```python
from build123d import *

# Parameters (mm, degrees)
F1_DEPTH       = 1.5
F2_DEPTH       = 10
F3_D           = 5
F3_CSINK_D     = 7
F3_CSINK_ANGLE = 90
F4_T1_DEPTH    = 36.6824583655
F4_T3_DEPTH    = 79.6824583655
F4_T5_DEPTH    = 19.5
F4_T7_DEPTH    = 47
F4_T13_DEPTH   = 52
F4_T17_DEPTH   = 24.5
F4_T24_DEPTH   = 24.5
F4_T28_DEPTH   = 52
F5_R           = 1


# Not quite as in the source:
# - a fillet or chamfer that OpenCascade refuses, or shapes differently, is made with other operations: its cross-section is extruded or revolved along the edge and cut away or added


with BuildPart() as f1:
    # F0 (on Front) → F1 (new body)
    with BuildSketch(Plane.XZ):
        Polygon((35, 27), (-35, 27), (-35, 0), (-25, 0), (-25, 16), (25, 16), (25, 0), (35, 0), align=None)
        Polygon((-25, 16), (-25, 0), (-23.5, 0), (-23.5, 14.5), (23.5, 14.5), (23.5, 0), (25, 0), (25, 16), align=None)
    extrude(amount=-F1_DEPTH)

    # F0 (on Front) → F2 (join)
    with BuildSketch(Plane.XZ):
        Polygon((-25, 16), (-25, 0), (-23.5, 0), (-23.5, 14.5), (23.5, 14.5), (23.5, 0), (25, 0), (25, 16), align=None)
    extrude(amount=-F2_DEPTH)

    # F3 (through all)
    with Locations(Plane.XZ):
        with Locations((28.6, 20.6), (-28.6, 20.6)):
            CounterSinkHole(F3_D / 2, F3_CSINK_D / 2, counter_sink_angle=F3_CSINK_ANGLE)

    # F4: fillet of radius 2 on 6 edges, made by hand

    # F4_s2 → F4_t1 (cut)
    with BuildSketch(Plane.XY.offset(-4.8412291828)):
        with BuildLine():
            ThreePointArc((-33.0635083269, 0), (-34.2882531983, 0.4188611699), (-35, 1.5))
            Line((-35, 1.5), (-35.0387298335, 1.49))
            ThreePointArc((-35.0387298335, 1.49), (-35.04, 0.75), (-35.04, 0))
            Line((-35.04, 0), (-35, -0.04))
            Line((-35, -0.04), (-33.0635083269, -0.04))
            Line((-33.0635083269, -0.04), (-33.0635083269, 0))
        make_face()
        with BuildLine():
            ThreePointArc((35, 1.5), (34.2882531983, 0.4188611699), (33.0635083269, 0))
            Line((33.0635083269, 0), (33.0635083269, -0.04))
            Line((33.0635083269, -0.04), (35, -0.04))
            Line((35, -0.04), (35.04, 0))
            ThreePointArc((35.04, 0), (35.04, 0.75), (35.0387298335, 1.49))
            Line((35.0387298335, 1.49), (35, 1.5))
        make_face()
    extrude(amount=F4_T1_DEPTH, mode=Mode.SUBTRACT)

    # F4_s4 → F4_t3 (cut)
    with BuildSketch(Plane.YZ.offset(-39.8412291828)):
        with BuildLine():
            ThreePointArc((1.5, 27), (0.4188611699, 26.2882531983), (0, 25.0635083269))
            Line((0, 25.0635083269), (-0.04, 25.0635083269))
            Line((-0.04, 25.0635083269), (-0.04, 27))
            Line((-0.04, 27), (0, 27.04))
            ThreePointArc((0, 27.04), (0.75, 27.04), (1.49, 27.0387298335))
            Line((1.49, 27.0387298335), (1.5, 27))
        make_face()
    extrude(amount=F4_T3_DEPTH, mode=Mode.SUBTRACT)

    # F4_s6 → F4_t5 (cut)
    with BuildSketch(Plane.XY.offset(-5)):
        with BuildLine():
            ThreePointArc((-25.5, 0), (-24.0857864376, 0.5857864376), (-23.5, 2))
            Line((-23.5, 2), (-23.46, 2))
            Line((-23.46, 2), (-23.46, -0.04))
            Line((-23.46, -0.04), (-25.5, -0.04))
            Line((-25.5, -0.04), (-25.5, 0))
        make_face()
        with BuildLine():
            ThreePointArc((25.5, 0), (24.0857864376, 0.5857864376), (23.5, 2))
            Line((23.5, 2), (23.46, 2))
            Line((23.46, 2), (23.46, -0.04))
            Line((23.46, -0.04), (25.5, -0.04))
            Line((25.5, -0.04), (25.5, 0))
        make_face()
    extrude(amount=F4_T5_DEPTH, mode=Mode.SUBTRACT)

    # F4_s8 → F4_t7 (cut)
    with BuildSketch(Plane.YZ.offset(-23.5)):
        with BuildLine():
            ThreePointArc((0, 16.5), (0.5857864376, 15.0857864376), (2, 14.5))
            Line((2, 14.5), (2, 14.46))
            Line((2, 14.46), (-0.04, 14.46))
            Line((-0.04, 14.46), (-0.04, 16.5))
            Line((-0.04, 16.5), (0, 16.5))
        make_face()
    extrude(amount=F4_T7_DEPTH, mode=Mode.SUBTRACT)


with BuildPart() as f4_tool11:
    # F4_s12 → F4_t13 (new body)
    with BuildSketch(Plane.YZ.offset(-28.5)):
        with BuildLine():
            ThreePointArc((0, 16.5), (0.5857864376, 15.0857864376), (2, 14.5))
            Line((2, 14.5), (2, 14.46))
            Line((2, 14.46), (-0.04, 14.46))
            Line((-0.04, 14.46), (-0.04, 16.5))
            Line((-0.04, 16.5), (0, 16.5))
        make_face()
    extrude(amount=F4_T13_DEPTH)

    split(bisect_by=Plane.YZ.offset(-23.5), keep=Keep.BOTTOM)


with BuildPart() as f4_tool15:
    # F4_s16 → F4_t17 (new body)
    with BuildSketch(Plane.XY.offset(-5)):
        with BuildLine():
            ThreePointArc((-25.5, 0), (-24.0857864376, 0.5857864376), (-23.5, 2))
            Line((-23.5, 2), (-23.46, 2))
            Line((-23.46, 2), (-23.46, -0.04))
            Line((-23.46, -0.04), (-25.5, -0.04))
            Line((-25.5, -0.04), (-25.5, 0))
        make_face()
    extrude(amount=F4_T17_DEPTH)

    split(bisect_by=Plane.XY.offset(14.5), keep=Keep.TOP)


with BuildPart() as f4_tool11_1:
    add(f4_tool11.part)

    # F4_t19: intersect F4_tool15
    add(f4_tool15.part, mode=Mode.INTERSECT)


with BuildPart() as f1_1:
    add(f1.part)

    # F4_t9: cut F4_tool11
    add(f4_tool11_1.part, mode=Mode.SUBTRACT)


with BuildPart() as f4_tool22:
    # F4_s23 → F4_t24 (new body)
    with BuildSketch(Plane.XY.offset(19.5)):
        with BuildLine():
            ThreePointArc((25.5, 0), (24.0857864376, 0.5857864376), (23.5, 2))
            Line((23.5, 2), (23.46, 2))
            Line((23.46, 2), (23.46, -0.04))
            Line((23.46, -0.04), (25.5, -0.04))
            Line((25.5, -0.04), (25.5, 0))
        make_face()
    extrude(amount=-F4_T24_DEPTH)

    split(bisect_by=Plane.XY.offset(14.5), keep=Keep.TOP)


with BuildPart() as f4_tool26:
    # F4_s27 → F4_t28 (new body)
    with BuildSketch(Plane.YZ.offset(-23.5)):
        with BuildLine():
            ThreePointArc((0, 16.5), (0.5857864376, 15.0857864376), (2, 14.5))
            Line((2, 14.5), (2, 14.46))
            Line((2, 14.46), (-0.04, 14.46))
            Line((-0.04, 14.46), (-0.04, 16.5))
            Line((-0.04, 16.5), (0, 16.5))
        make_face()
    extrude(amount=F4_T28_DEPTH)

    split(bisect_by=Plane.YZ.offset(23.5), keep=Keep.TOP)


with BuildPart() as f4_tool22_1:
    add(f4_tool22.part)

    # F4_t30: intersect F4_tool26
    add(f4_tool26.part, mode=Mode.INTERSECT)


with BuildPart() as f1_2:
    add(f1_1.part)

    # F4_t20: cut F4_tool22
    add(f4_tool22_1.part, mode=Mode.SUBTRACT)

    # F5
    f5_edges = [f1_2.edges().sort_by_distance(p)[0] for p in [
        (25, 1.5, 8),
        (0, 1.5, 16),
        (-25, 1.5, 8),
    ]]
    fillet(f5_edges, radius=F5_R)


solid = f1_2.part
```
Check sheet for the modelled part. Datum: model origin and axes. Units: mm. A direction names the side the tool comes from. Round coordinates to 2 decimals unless told otherwise and drop trailing zeros. Write each loop counter-clockwise with the first axis right and the second up, starting at its lowest first coordinate (ties: lowest second). Pieces come first, ordered by that corner, then holes. Notation, with made-up numbers: M 73,28.5 L 116,28.5 A23 ccw 116,56.5 Z; hole C 26,0.25 d6. An arc over 180 degrees is marked long. Write item = value, one per line. Start each with the question number.
1. Section check C-C, the plane z = 20.6. Record the cut outline in (x, y), then the cut area to 3 significant figures.
2. Tool access check on faces 4 (the flat face through (-25, 6, 8)), 5 (the cylindrical face through (-0.36, 0.57, 15.1)), 6 (the flat face through (-23.5, 6, 7)), 7 (the flat face through (25, 6, 8)). Record the directions out of +Z, -Z, +X, -X, +Y, -Y that give a thin tool (end or side, any length) a straight path to the whole face; none if there is none.
3. Section check A-A, the plane x = 28.6. Record the cut outline in (y, z), then the cut area to 3 significant figures.
4. Gauge pin test, flat ends, axial feed: pin 1 (4 mm diameter, centred on y = 5, z = 11.5, fed in from +X); pin 2 (4.5 mm diameter, centred on x = 28.6, z = 20.6, fed in from -Y); pin 3 (6.5 mm diameter, centred on x = -28.6, z = 20.6, fed in from -Y); pin 4 (6 mm diameter, centred on x = -11, y = 1.5, fed in from -Z). Record the tip position at first contact, or that the pin passes through.
5. Section check B-B, the plane z = 4. Record the cut outline in (x, y).
6. Scan lines: line 1 (X direction, y = 1.45, z = 20.6); line 2 (X direction, y = 1.1, z = 20.6); line 3 (Z direction, x = -28.6, y = 1.45). Record each from-to range of solid material in increasing order. Write a range as [from, to].
7. Section check D-D, the plane y = 8. Record the cut outline in (x, z).
8. Release check for a two-part mould opening along Z. For faces 1 (the flat face through (0, 6, 14.5)), 2 (the cylindrical face through (-30.91, 1.25, 19.64)), 3 (the cylindrical face through (-0.49, 0.43, 26.3)) record: pulls with the +Z half, pulls with the -Z half, needs draft (parallel to the pull), parting line crosses it, or undercut.
Results found:
q1.outline = M -35,1.5 A2 ccw -33.06,0 L -32.1,0 L -31.1,1 L -31.1,1.5 Z; M -26.1,1 L -25.1,0 L 25.1,0 L 26.1,1 L 26.1,1.5 L -26.1,1.5 Z; M 31.1,1 L 32.1,0 L 33.06,0 A2 ccw 35,1.5 L 31.1,1.5 Z
q1.area = 86.5 mm^2
q2.face_4 = +Z, -Z, -X, +Y
q2.face_5 = -Z, -Y
q2.face_6 = -Z, +Y, -Y
q2.face_7 = +Z, -Z, +X, +Y
q3.outline = M 0,0 L 1.5,0 L 1.5,18.1 L 1,18.1 L 0,17.1 Z; M 0,24.1 L 1,23.1 L 1.5,23.1 L 1.5,27 A2 ccw 0,25.06 Z
q3.area = 31.2 mm^2
q4.pin_1 = 25
q4.pin_2 = through
q4.pin_3 = 0.25
q4.pin_4 = 14.5
q5.outline = M -35,1.5 A2 ccw -33.06,0 L -25.5,0 A2 ccw -23.5,2 L -23.5,10 L -25,10 L -25,2.5 A1 cw -26,1.5 Z; M 23.5,2 A2 ccw 25.5,0 L 33.06,0 A2 ccw 35,1.5 L 26,1.5 A1 cw 25,2.5 L 25,10 L 23.5,10 Z
q6.line_1 = [-34.99, -31.1], [-26.1, 26.1], [31.1, 34.99]
q6.line_2 = [-34.85, -31.1], [-26.1, 26.1], [31.1, 34.85]
q6.line_3 = [0, 18.1], [23.1, 26.99]
q7.outline = M -25,0 L -23.5,0 L -23.5,14.5 L 23.5,14.5 L 23.5,0 L 25,0 L 25,16 L -25,16 Z
q8.face_1 = pulls with the -Z half
q8.face_2 = undercut
q8.face_3 = pulls with the +Z half
